Input: part model. Units: mm. Frame: model coordinates. Face numbers are marked on the shaded views. A direction names the side the tool comes from. Round coordinates to 2 decimals unless told otherwise and drop trailing zeros. Loops run counter-clockwise (first coordinate to the right, second up) from the corner with the lowest first, then second, coordinate; pieces in that order, holes last. Notation, with made-up numbers: M -33.5,59 L -0.5,59 A34 cw -0.5,96 Z; hole C 58.5,-30.5 d3. An arc over 180 degrees is marked long. Use one line per item in the form item = value. Start each with the question number.
Q1. Section query B-B, the plane x = 0. Output: boundary loops of the cut face in (y, z).
Q2. First-contact query: P1, Ø1.4, axis at x = 24, y = -5, coming from the -Z side. Flat tip, straight axial feed; report the tip coordinate or a pass-through.
Q3. Mould query, pull axis X, two halves, no side actions, for the marked faces 1, 2, 3 and 4. Classes: pulls with the +X half, pulls with the -X half, needs draft (parallel to the pull), parting line crosses it, or undercut.
Q4. Ray query, line 1 along Y through (x, z) = (24, 1.05); line 2 along X through (y, z) = (-3, 10.75); line 3 along Z through (x, y) = (25.5, -3.25). Return the intervals inside material, ascending.
Q5. Section query A-A, the plane z = 1. Output: boundary loops of the cut face in (x, y), and give its area (3 significant figures).
Q6. Access query for the marked faces 5, 6 and 7. Directions: +Z, -Z, +X, -X, +Y, -Y. A direction counts if a zero-diameter tool reaches every point of the face in a straight line with its end or side. Return the directions, or none.
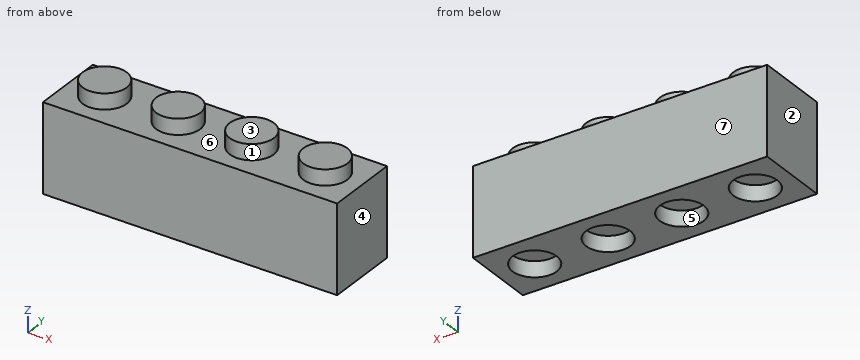
```python
from build123d import *

# Parameters (mm, degrees)
F1_DEPTH = 8
F3_W     = 8
F3_H     = 8
F3_R     = 2.4
F4_DEPTH = 1.7
F5_R     = 2.4
F6_DEPTH = 1.7


with BuildPart() as f1:
    # F0 (on Front) → F1 (new body)
    with BuildSketch(Plane.XZ):
        Polygon((-2.4, 9.6), (-4, 9.6), (-4, 0), (4, 0), (4, 9.6), (2.4, 9.6), (2.4, 11.3), (-2.4, 11.3), align=None)
    extrude(amount=F1_DEPTH)

    # F3 (on plane+point) → F4 (cut, through all)
    with BuildSketch(Plane.XY.offset(11.3)):
        with Locations((0, -4)):
            Rectangle(F3_W, F3_H)
        with Locations((0, -4)):
            Circle(F3_R, mode=Mode.SUBTRACT)
    extrude(amount=-F4_DEPTH, mode=Mode.SUBTRACT)

    # F5 (on Top) → F6 (cut)
    with BuildSketch(Plane.XY):
        with Locations((0, -4)):
            Circle(F5_R)
    extrude(amount=F6_DEPTH, mode=Mode.SUBTRACT)

    # F8: F1 across plane


with BuildPart() as f1_1:
    add(f1.part)
    add(f1.part.mirror(Plane.YZ.offset(4)))

    # F10: F1 across plane


with BuildPart() as f1_2:
    add(f1_1.part)
    add(f1_1.part.mirror(Plane.YZ.offset(12)))


solid = f1_2.part
```
Results found:
q1.outline = M -8,0 L -6.4,0 L -6.4,1.7 L -1.6,1.7 L -1.6,0 L 0,0 L 0,9.6 L -1.6,9.6 L -1.6,11.3 L -6.4,11.3 L -6.4,9.6 L -8,9.6 Z
q2.P1 = 1.7
q3.face_1 = undercut
q3.face_2 = pulls with the -X half
q3.face_3 = needs draft
q3.face_4 = pulls with the +X half
q4.line_1 = -8 to -6.4, -1.6 to 0
q4.line_2 = -2.18 to 2.18, 5.82 to 10.18, 13.82 to 18.18, 21.82 to 26.18
q4.line_3 = 1.7 to 11.3
q5.outline = M -4,-8 L 28,-8 L 28,0 L -4,0 Z; hole C 0,-4 d4.8; hole C 8,-4 d4.8; hole C 16,-4 d4.8; hole C 24,-4 d4.8
q5.area = 184 mm²
q6.face_5 = -Z
q6.face_6 = +Z
q6.face_7 = +Z, -Z, +X, -X, +Y
